Can you work these out from the model? Positions are in its coordinate system, mm. Face numbers are marked on the shaded views. A direction names the side the tool comes from. Give positions to 0.01 mm unless a question says otherwise; leave off trailing zeros. Write each loop counter-clockwise with the first axis right and the second up, starting at its lowest first coordinate (ties: lowest second). Pieces come first, ordered by that corner, then holes.
from build123d import *

# Parameters (mm, degrees)
F0_W     = 43
F0_H     = 43
F1_DEPTH = 1.5
F2_W     = 23
F2_H     = 16
F3_DEPTH = 25
F4_R     = 1.5
F5_DEPTH = 1.501


with BuildPart() as f1:
    # F0 (on Top) → F1 (new body)
    with BuildSketch(Plane.XY):
        Rectangle(F0_W, F0_H)
    extrude(amount=F1_DEPTH)

    # F2 (on face) → F3 (join)
    with BuildSketch(Plane.XY.offset(1.5)):
        with Locations((0, -13.5)):
            Rectangle(F2_W, F2_H)
    extrude(amount=F3_DEPTH)

    # F4 (on face) → F5 (cut, through all)
    with BuildSketch(Plane.XY.offset(1.5)):
        with Locations((-19, -19)):
            Circle(F4_R)
        with Locations((19, -19)):
            Circle(F4_R)
        with Locations((-19, 19)):
            Circle(F4_R)
        with Locations((19, 19)):
            Circle(F4_R)
    extrude(amount=-F5_DEPTH, mode=Mode.SUBTRACT)


solid = f1.part
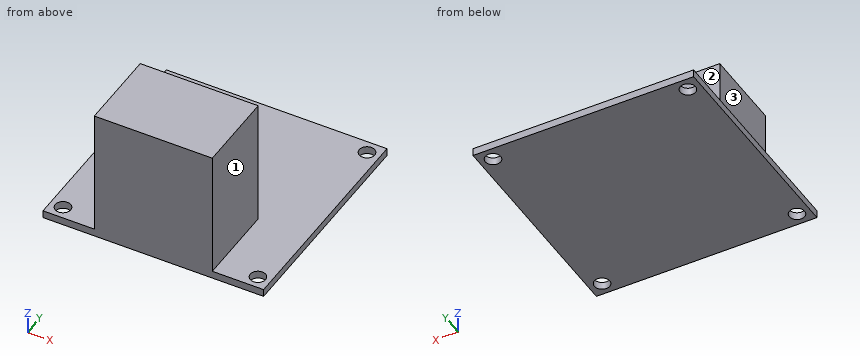
(1) Imagine slicing it at C-C, the plane x = -1. Write out the boundary of the cut face in (y, z), plus the area to 4 significant figures.
Returned:
outline: (-21.5, 0) - (21.5, 0) - (21.5, 1.5) - (-5.5, 1.5) - (-5.5, 26.5) - (-21.5, 26.5) - close
area: 464.5 mm2
(2) Imagine slicing it at D-D, the plane y = -12.5. Write out the boundary of the cut face in (x, z), plus the area to 4 significant figures.
Returned:
outline: (-21.5, 0) - (21.5, 0) - (21.5, 1.5) - (11.5, 1.5) - (11.5, 26.5) - (-11.5, 26.5) - (-11.5, 1.5) - (-21.5, 1.5) - close
area: 639.5 mm2
(3) Will these pins go through, and if not, where does the flat tip stop? P1, Ø6, axis at y = -11.5, z = 16, coming from the -X side; P2, Ø5, axis at y = -15, z = 10.5, coming from the +X side; P3, Ø1, axis at x = -1, z = 21, coming from the +Y side.
Returned:
P1: stops at x = -11.5
P2: stops at x = 11.5
P3: stops at y = -5.5
(4) If I drill on L1, parallel to Y at x = 19, z = 0.6; L2, parallel to X at y = -10, z = 24; L3, parallel to Y at x = -1.5, z = 21.75, over which ranges is the centre line in solid material (lowest first)?
Returned:
L1: y = -21.5 to -20.5, -17.5 to 17.5, 20.5 to 21.5
L2: x = -11.5 to 11.5
L3: y = -21.5 to -5.5
(5) For the marked faces 1, 2 and 3, which set-ups out of +Z, -Z, +X, -X, +Y, -Y let a thin tool reach every point of the face, with its end or its side?
Returned:
face 1: +Z, +X, +Y, -Y
face 2: +Z, +X, -X, +Y
face 3: +Z, -X, +Y, -Y
(6) Imagine slicing it at A-A, the plane x = -19. Write out the boundary of the cut face in (y, z).
Returned:
outline: (-21.5, 0) - (-20.5, 0) - (-20.5, 1.5) - (-21.5, 1.5) - close; (-17.5, 0) - (17.5, 0) - (17.5, 1.5) - (-17.5, 1.5) - close; (20.5, 0) - (21.5, 0) - (21.5, 1.5) - (20.5, 1.5) - close
